Work out the finished part from the listing and answer in its coordinate system (mm). A direction names the side the tool comes from. Give positions to 0.01 mm unless a question says otherwise; leave off trailing zeros. Loops run counter-clockwise (first coordinate to the right, second up) from the corner with the lowest first, then second, coordinate; pieces in that order, holes last. Notation, with made-up numbers: (19.5, -30.75) -> (73.5, -30.75) arc R16 ccw to (73.5, -7.75) -> close; hole circle Ø5 at (7.25, 40). An arc over 180 degrees is marked (long way). Answer as CSV lines item,"result". Start each with the question number.
1. Find section C-C, the plane x = -3.25. Give the vertices of the cut face in (y, z).
2. Find section B-B, the plane y = 8. Give the vertices of the cut face in (x, z), and give its area (3 significant figures).
3. Flat-ended cylindrical pins translate along their axes: pin 1 Ø5.5 at (x, z) = (0.53, 114.3) entering from -Y; pin 2 Ø8 at (x, y) = (7.5, 9.5) entering from +Z. Find the tip coordinate at first contact, or state that the pin passes through.
4. Determine the mould class of faces 3 (the face through (-2, -33.523, 63)), 4 (the face through (12.603, -8.765, 58.724)), 5 (the face through (13.229, -9, 63)) for opening direction X: +X half, -X half, draft (parallel to the pull), parting line (faces both ways), or undercut.
5. Find section A-A, the plane z = 63.5. Give the vertices of the cut face in (x, y), and give its area (3 significant figures).
6. Find section D-D, the plane z = 98. Give the vertices of the cut face in (x, y), and give its area (3 significant figures).
7. Find the intervals of material crossed by line 1 along Y through (x, z) = (-11.2, 44.45); line 2 along Y through (x, z) = (1.75, 18.5); line 3 along X through (y, z) = (0, 18.5), in increasing order.
8. A tool of negligible diameter and unlimited length cuts with its end or side. For faces 1 (the face through (-10.901, -9, 63)), 2 (the face through (0.3, 15.38, 36.39)), from which of +Z, -Z, +X, -X, +Y, -Y can it reach the whole face along a straight path? Write none if from no direction.
Autodesk Inventor part; units mm, degrees
ref_plane "YZ Plane" through (0, 0, 0) normal (1, 0, 0) x (0, 1, 0)
ref_plane "XZ Plane" through (0, 0, 0) normal (0, 1, 0) x (-1, 0, 0)
ref_plane "XY Plane" through (0, 0, 0) normal (0, 0, 1) x (1, 0, 0)
sketch "Sketch1" plane through (0, 0, 0) normal (0, 0, 1) x (1, 0, 0)
  line L0 (-12.1708, 16.0073) -> (13.2292, 16.0073)
  line L1 (13.2292, 16.0073) -> (13.2292, -34.7927)
  line L2 (13.2292, -34.7927) -> (-12.1708, -34.7927)
  line L3 (-12.1708, -34.7927) -> (-12.1708, 16.0073)
  line L4 (11.9592, 14.7373) -> (-10.9008, 14.7373)
  line L5 (-10.9008, 14.7373) -> (-10.9008, -33.5227)
  line L6 (-10.9008, -33.5227) -> (11.9592, -33.5227)
  line L7 (11.9592, -33.5227) -> (11.9592, 14.7373)
  point P0 (0, 0)
  dimension "d0" = 25.4
  dimension "d1" = 50.8
  dimension "d2" = 1.27
extrude "Extrusion1" add sketch "Sketch1" along normal blind 127
sketch "Sketch2" plane through (-12.1708, 16.0073, 0) normal (0, 1, 0) x (1, 0, 0)
  circle A0 centre (12.7, -12.7) radius 1.7272
  line L0 (25.4, 0) -> (0, 0)
  line L1 (0, 0) -> (0, -127)
  point P0 (12.1708, 0)
  dimension "d5" = 3.4544
  dimension "d6" = 12.7
  dimension "d7" = 12.7
extrude "Extrusion2" cut sketch "Sketch2" against normal through all
pattern_linear "Rectangular Pattern1" count 13 spacing 25.4 along (0, 0, 1) of "Extrusion2"
sketch "Sketch3" plane through (13.2292, -34.7927, 0) normal (1, 0, 0) x (0, 0, -1)
  circle A0 centre (-44.45, 25.4) radius 14.2875
  line L0 (-127, 0) -> (-127, 50.8)
  line L1 (0, 0) -> (0, 50.8)
  line L2 (0, 50.8) -> (-127, 50.8)
  point P0 (0, 34.7927)
  dimension "d15" = 28.575
  dimension "d18" = 25.4
  dimension "d21" = 44.45
extrude "Extrusion3" cut sketch "Sketch3" against normal blind 25.4
equation "\"d3\" = d13"
equation "\"d10\" = d14"
equation "\"d13\" = 127"
equation "\"d14\" = d13"
properties part number "RailSupp"
Resolved:
1,outline,"(-34.79, 0) -> (-33.52, 0) -> (-33.52, 127) -> (-34.79, 127) -> close; (14.74, 0) -> (16.01, 0) -> (16.01, 127) -> (14.74, 127) -> close"
2,outline,"(-12.17, 0) -> (-10.9, 0) -> (-10.9, 127) -> (-12.17, 127) -> close; (11.96, 0) -> (13.23, 0) -> (13.23, 127) -> (11.96, 127) -> close"
2,area,"323 mm^2"
3,pin 1,"stops at y = -34.79"
3,pin 2,"passes through"
4,face 3,"undercut"
4,face 4,"draft"
4,face 5,"+X half"
5,outline,"(-12.17, -34.79) -> (-1.2, -34.79) -> (-1.2, -33.52) -> (-10.9, -33.52) -> (-10.9, 14.74) -> (-1.2, 14.74) -> (-1.2, 16.01) -> (-12.17, 16.01) -> close; (2.26, -34.79) -> (13.23, -34.79) -> (13.23, 16.01) -> (2.26, 16.01) -> (2.26, 14.74) -> (11.96, 14.74) -> (11.96, -33.52) -> (2.26, -33.52) -> close"
5,area,"178 mm^2"
6,outline,"(-12.17, -34.79) -> (13.23, -34.79) -> (13.23, 16.01) -> (-12.17, 16.01) -> close; hole (-10.9, -33.52) -> (11.96, -33.52) -> (11.96, 14.74) -> (-10.9, 14.74) -> close"
6,area,"187 mm^2"
7,line 1,"y = -34.79 to -23.68, 4.89 to 16.01"
7,line 2,"y = -34.79 to -33.52, 14.74 to 16.01"
7,line 3,"x = -12.17 to -10.9, 11.96 to 13.23"
8,face 1,"+Z, -Z"
8,face 2,"+Y, -Y"
